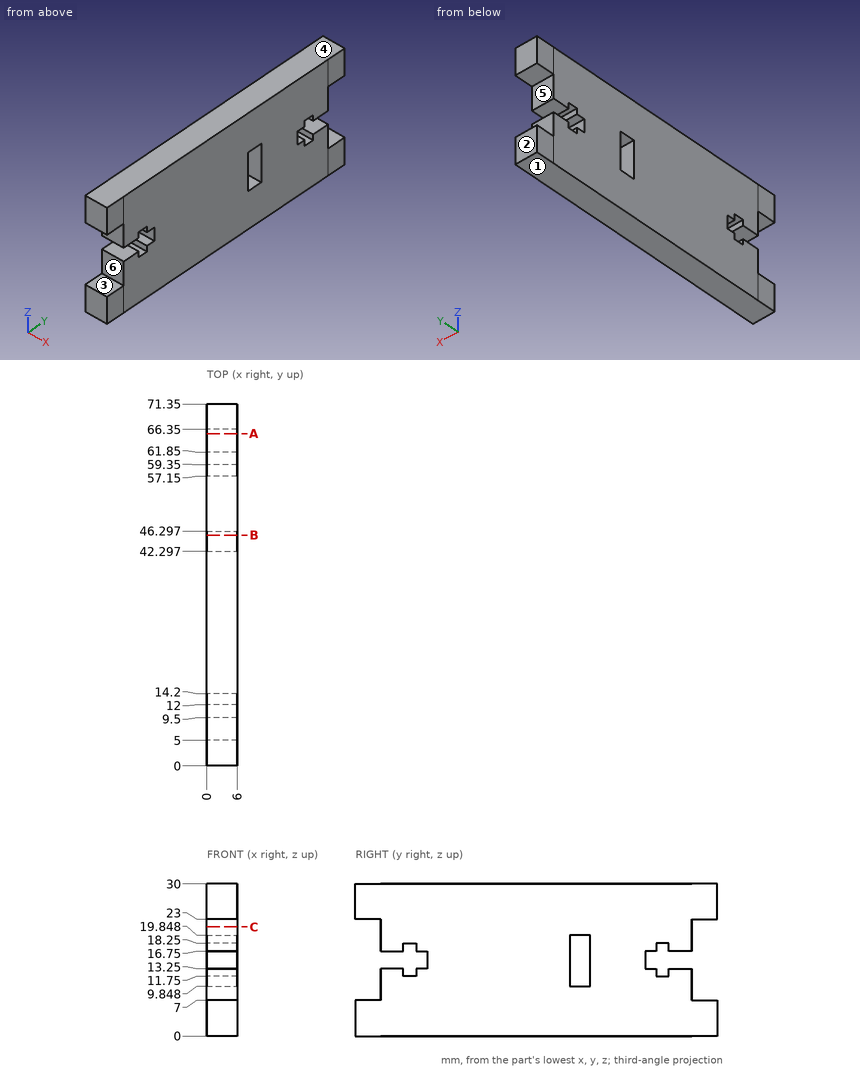
Verification items for this drawing (mm, ordinates from the low corner). A direction names the side the tool comes from. Coordinates: 2 decimals unless noted, no trailing zeros. Write each loop counter-clockwise with the first axis right and the second up, starting at its lowest first coordinate (ties: lowest second). Pieces come first, ordered by that corner, then holes. Notation, with made-up numbers: M -14.5,-14.5 L 34.5,-14.5 A6 cw 34.5,-10.5 Z; hole C 81.25,13 d5. An arc over 180 degrees is marked long. Answer as a JSON object with one key per item and string values. Group by question number.
(1) Cross-section at C-C, the plane z = 21.5. Record the cut outline in (x, y), and give its area (3 significant figures).
(2) Cross-section at B-B, the plane y = 45.5. Record the cut outline in (x, z), and give its area (3 significant figures).
(3) Material ranges on line 1 (Y direction, x = 4, z = 17); line 2 (Y direction, x = 0.5, z = 15.25); line 3 (Z direction, x = 1, y = 3), recorded low to high.
(4) Cross-section at A-A, the plane y = 65.5. Record the cut outline in (x, z).
(5) Release check for a two-part mould opening along Z. For the marked faces 1, 2 and 3 record: +Z half, -Z half, draft (parallel to the pull), parting line (faces both ways), or undercut.
(6) Tool access check on the marked faces 4, 5 and 6. Record the directions out of +Z, -Z, +X, -X, +Y, -Y that give a thin tool (end or side, any length) a straight path to the whole face; none if there is none.
(7) Gauge pin test, flat end, axial feed: pin 1 (1.8 mm diameter, centred on x = 2.5, z = 13.5, fed in from +Y). Record the tip position at first contact, or that the pin passes through.
Reply:
{
 "1": {"outline": "M 0,5 L 6,5 L 6,66.35 L 0,66.35 Z", "area": "368 mm²"},
 "2": {"outline": "M 0,0 L 6,0 L 6,9.85 L 0,9.85 Z; M 0,19.85 L 6,19.85 L 6,30 L 0,30 Z", "area": "120 mm²"},
 "3": {"line 1": "5 to 9.5, 12 to 42.3, 46.3 to 59.35, 61.85 to 66.35", "line 2": "14.2 to 42.3, 46.3 to 57.15", "line 3": "0 to 7, 23 to 30"},
 "4": {"outline": "M 0,0 L 6,0 L 6,13.25 L 0,13.25 Z; M 0,16.75 L 6,16.75 L 6,30 L 0,30 Z"},
 "5": {"face 1": "-Z half", "face 2": "draft", "face 3": "undercut"},
 "6": {"face 4": "+Z, +X, -X, +Y, -Y", "face 5": "+X, -X, +Y", "face 6": "+X, -X, -Y"},
 "7": {"pin 1": "y = 66.35"}
}
